Read the model definition and answer for the solid it produces. Units are mm, in the model's axes. Coordinates: 2 decimals unless noted, no trailing zeros. Write each loop counter-clockwise with the first axis right and the second up, starting at its lowest first coordinate (ties: lowest second). Pieces come first, ordered by that corner, then holes. Notation, with made-up numbers: (15.25, 35) -> (24.25, 35) arc R16 cw to (24.25, 63) -> close; hole circle Ø2 at (-2.75, -38.5). An arc over 180 degrees is marked (long way). One line per item, written item: value. Start each with the question number.
1. Consider line 1 along Y through (x, z) = (1.55, 0); line 2 along X through (y, z) = (20, -6); line 3 along Z through (x, y) = (5.5, 4) (3 decimals). Determine where each line is inside the solid, lowest interval first.
2. Given P1, Ø11.5, axis at y = 14.5, z = -2.5, coming from the +X side; P2, Ø3.5, axis at x = 5, z = 15.5, coming from the +Y side; P3, Ø0.9, axis at x = 4, y = -5, coming from the +Z side, each flat-ended and moving along its own axis, determine where each tip first touches the part or whether it passes through.
3. Find section C-C, the plane z = 33. Write down the section's boundary in (x, y), and give its area (3 significant figures).
4. Find section B-B, the plane y = 1. Write down the section's boundary in (x, z) (3 decimals).
5. Find section A-A, the plane z = 0. Write down the section's boundary in (x, y), and give its area (3 significant figures).
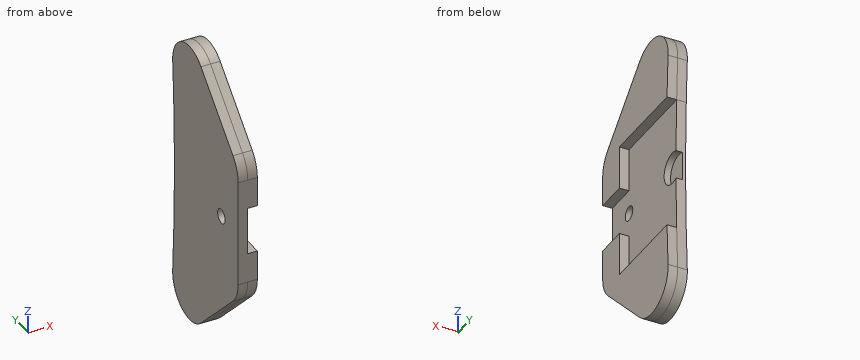
Autodesk Inventor part; units mm, degrees
ref_plane "YZ Plane" through (0, 0, 0) normal (1, 0, 0) x (0, 1, 0)
ref_plane "XZ Plane" through (0, 0, 0) normal (0, 1, 0) x (-1, 0, 0)
ref_plane "XY Plane" through (0, 0, 0) normal (0, 0, 1) x (1, 0, 0)
sketch "Sketch1" plane through (0, 0, 0) normal (1, 0, 0) x (0, 1, 0)
  line L0 (10, 21.125) -> (-10, 21.125)
  line L1 (-10, 21.125) -> (-10, -21.125)
  line L2 (-10, -21.125) -> (10, -21.125)
  line L3 (10, -21.125) -> (10, 21.125)
  line L4 (10, 21.125) -> (-10, -21.125) construction
  line L5 (-10, 21.125) -> (10, -21.125) construction
  point P0 (0, 0)
  dimension "d0" = 42.25
  dimension "d1" = 20
extrude "Extrusion1" add sketch "Sketch1" along normal blind 6
sketch "Sketch2" plane through (6, 0, 0) normal (1, 0, 0) x (0, 0, -1)
  line L0 (-21.125, 0) -> (-7.5, 0)
  line L1 (-7.5, 0) -> (-7.5, -10)
  line L2 (-21.125, -10) -> (21.125, -10)
  line L3 (7.5, 0) -> (21.125, 0)
  line L4 (21.125, -10) -> (21.125, 10)
  line L5 (7.5, 0) -> (7.5, -10.6285)
  line L6 (-21.125, -10) -> (21.125, -10)
  line L7 (21.125, -10) -> (21.125, 10)
  line L8 (21.125, 10) -> (-21.125, 10)
  line L9 (-21.125, 10) -> (-21.125, -10)
  point P0 (0, 0)
  point P1 (0, -10)
  point P2 (-21.125, 0)
  point P3 (7.5, -10)
  dimension "d4" = 15
  dimension "d6" = 10
  dimension "d7" = 7.5
extrude "Extrusion2" cut sketch "Sketch2" against normal blind 3 contours L9 L8 L4 L3 L5 L2 L1 L0
sketch "Sketch4" plane through (0, 0, 0) normal (-1, 0, 0) x (0, 0, 1)
  arc A0 (21.125, 28.5) -> (190.4596, 58.7605) centre (0, 635.6334) ccw
  circle A1 centre (0, 635.6334) radius 607.5008
  circle A2 centre (0, 635.6334) radius 607.5008
  circle A3 centre (0, 635.6334) radius 617.5008
  line L0 (21.125, 0) -> (21.125, -10)
  line L1 (21.125, -10) -> (50, 20.1602)
  line L2 (-7.5, -10) -> (-21.125, -10)
  line L3 (-21.125, -10) -> (-50, 20.1602)
  line L4 (-50, 20.1602) -> (-50, 30.1937)
  line L5 (50, 20.1602) -> (50, 30.1937)
  line L6 (21.125, -10) -> (-21.125, -10)
  point P0 (0, 0)
  dimension "d17" = 0
  dimension "d18" = 10
  dimension "d19" = 100
extrude "Extrusion3" add sketch "Sketch4" against normal blind 3 contours A0 L5 A3 L4 A1 | L1 L6 L2 L3 A3 picked at (-31.0009, 22.4071)
fillet "Fillet1" radius 10 4 edges at (1.5, 20.1602, 50) (1.5, 20.1602, -50) (1.5, 30.1937, -50) (1.5, 30.1937, 50)
sketch "Sketch3" plane through (3, 0, 0) normal (1, 0, 0) x (0, 0, -1)
  point P0 (0, 0)
  point P1 (0, 0)
  point P2 (7.5, 0)
hole "Hole1" at (3, 0, 0) direction (-1, 0, 0) diameter 4.5 end through all
sketch "Sketch5" plane through (3, 0, 0) normal (1, 0, 0) x (0, 0, -1)
  line L0 (-21.125, -10) -> (-7.5, -10)
  line L1 (-21.125, -10) -> (21.125, -10)
  line L2 (21.125, -10) -> (21.125, 40)
  line L3 (21.125, 40) -> (-21.125, 40)
  line L4 (-21.125, 40) -> (-21.125, -10)
  arc A0 (-34.605, 29.119) -> (-42.3979, 12.2197) centre (-35.1746, 19.1352) ccw
  line L5 (-42.3979, 12.2197) -> (-21.125, -10)
  line L6 (-21.125, 0) -> (-21.125, -10)
  line L7 (-7.5, 0) -> (-21.125, 0)
  line L8 (-7.5, -10) -> (-7.5, 0)
  line L9 (7.5, -10) -> (-7.5, -10)
  line L10 (7.5, 0) -> (7.5, -10)
  line L11 (21.125, 0) -> (7.5, 0)
  line L12 (21.125, -10) -> (21.125, 0)
  line L13 (21.125, -10) -> (42.3979, 12.2197)
  arc A1 (42.3979, 12.2197) -> (34.605, 29.119) centre (35.1746, 19.1352) ccw
  arc A2 (-34.605, 29.119) -> (34.605, 29.119) centre (0, 635.6334) ccw
  circle A3 centre (0, 0) radius 2.25
  point P0 (21.125, 28.5)
  point P1 (-21.125, 28.5)
  dimension "d26" = 50
extrude "Extrusion4" add sketch "Sketch5" along normal up to surface (3 mm away) contours L5 A0 A2 L4 | L2 A2 A1 L13
sketch "Sketch6" plane through (3, 0, 0) normal (1, 0, 0) x (0, 0, -1)
  circle A0 centre (0, 26) radius 5
  point P0 (0, 0)
  dimension "d27" = 26
  dimension "d28" = 10
extrude "Extrusion5" cut sketch "Sketch6" against normal blind 2
fillet "Fillet2" radius 10 2 edges at (3, -10, -21.125) (3, -10, 21.125)
properties part number "base_cover_3DPrint"
Answer block:
1. line 1: y = -10 to -2.25, 2.25 to 21
1. line 2: x = 0 to 3
1. line 3: z = -34.528 to -21.125, 21.125 to 34.528
2. P1: stops at x = 3
2. P2: stops at y = 0
2. P3: stops at z = 26.34
3. outline: (0, 2.4) -> (6, 2.4) -> (6, 29.03) -> (0, 29.03) -> close
3. area: 160 mm2
4. outline: (0, -31.656) -> (6, -31.656) -> (6, -21.125) -> (3, -21.125) -> (3, -2.016) -> (0, -2.016) -> close; (0, 2.016) -> (3, 2.016) -> (3, 21.125) -> (6, 21.125) -> (6, 31.656) -> (0, 31.656) -> close
5. outline: (0, -10) -> (3, -10) -> (3, -2.25) -> (0, -2.25) -> close; (0, 2.25) -> (3, 2.25) -> (3, 21) -> (1, 21) -> (1, 28.13) -> (0, 28.13) -> close
5. area: 86.6 mm2
